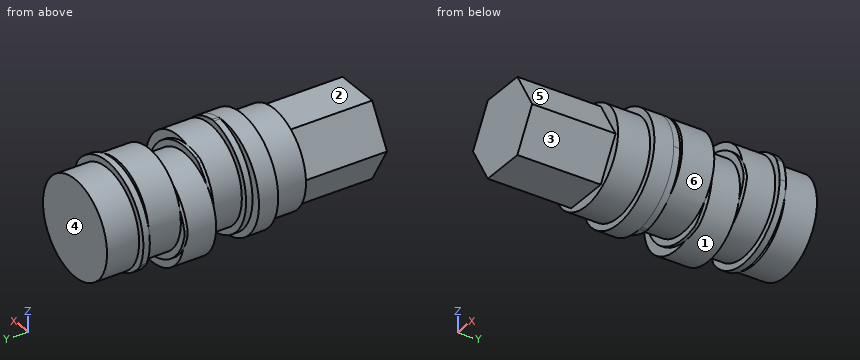
from build123d import *

# Parameters (mm, degrees)
BOSS_EXTRUDE1_DEPTH  = 13
SKETCH5_R            = 7.5
BOSS_EXTRUDE2_DEPTH  = 8
BOSS_EXTRUDE3_DEPTH  = 1
SKETCH7_R            = 7.5
BOSS_EXTRUDE4_DEPTH  = 5
BOSS_EXTRUDE5_DEPTH  = 0.5
SKETCH9_R            = 7.5
BOSS_EXTRUDE6_DEPTH  = 5
BOSS_EXTRUDE7_DEPTH  = 0.5
SKETCH12_R           = 7.5
BOSS_EXTRUDE8_DEPTH  = 5
BOSS_EXTRUDE9_DEPTH  = 1
SKETCH14_R           = 7.5
BOSS_EXTRUDE10_DEPTH = 5
FILLET1_R            = 2
BOSS_EXTRUDE11_START = 3
SKETCH15_R           = 8.5
BOSS_EXTRUDE11_DEPTH = 3


with BuildPart() as part:
    # Sketch4 → Boss-Extrude1 (new body)
    with BuildSketch(Plane(origin=(0, 0, 0), x_dir=(1, 0, 0), z_dir=(0, 1, 0))):
        Polygon((-3.464101615, 6), (-6.92820323, 0), (-3.464101615, -6), (3.464101615, -6), (6.92820323, 0), (3.464101615, 6), align=None)
    extrude(amount=BOSS_EXTRUDE1_DEPTH)

    # Sketch5 → Boss-Extrude2 (add)
    with BuildSketch(Plane(origin=(0, 13, 0), x_dir=(1, 0, 0), z_dir=(0, 1, 0))):
        with Locations(Location((0, 0, 0), (0, 0, 270))):
            Circle(SKETCH5_R)
    extrude(amount=BOSS_EXTRUDE2_DEPTH)

    # Sketch6 → Boss-Extrude3 (add)
    with BuildSketch(Plane(origin=(0, 21, 0), x_dir=(1, 0, 0), z_dir=(0, 1, 0))):
        with BuildLine():
            ThreePointArc((0.75, -8.466847111), (6.269968102, -5.739120142), (8.5, 0))
            ThreePointArc((8.5, 0), (6.269968102, 5.739120142), (0.75, 8.466847111))
            ThreePointArc((0.75, 8.466847111), (-7, 0), (0.75, -8.466847111))
        make_face()
    extrude(amount=BOSS_EXTRUDE3_DEPTH)

    # Sketch7 → Boss-Extrude4 (add)
    with BuildSketch(Plane(origin=(0, 22, 0), x_dir=(1, 0, 0), z_dir=(0, 1, 0))):
        with Locations(Location((1.5, 0, 0), (0, 0, 52.330113036))):
            Circle(SKETCH7_R)
    extrude(amount=BOSS_EXTRUDE4_DEPTH)

    # Sketch8 → Boss-Extrude5 (add)
    with BuildSketch(Plane(origin=(0, 27, 0), x_dir=(1, 0, 0), z_dir=(0, 1, 0))):
        with BuildLine():
            ThreePointArc((7.75, 1.299038106), (6.915283179, 4.972379062), (4.575074404, 7.924261316))
            ThreePointArc((4.575074404, 7.924261316), (-5.861215932, 4.25), (-3.825074404, -6.625223211))
            ThreePointArc((-3.825074404, -6.625223211), (4.051659482, -5.714810069), (7.75, 1.299038106))
        make_face()
    extrude(amount=BOSS_EXTRUDE5_DEPTH)

    # Sketch9 → Boss-Extrude6 (add)
    with BuildSketch(Plane(origin=(0, 27.5, 0), x_dir=(1, 0, 0), z_dir=(0, 1, 0))):
        with Locations(Location((-0.75, 1.299038106, 0), (0, 0, 73.730489259))):
            Circle(SKETCH9_R)
    extrude(amount=BOSS_EXTRUDE6_DEPTH)

    # Sketch11 → Boss-Extrude7 (add)
    with BuildSketch(Plane(origin=(0, 32.5, 0), x_dir=(1, 0, 0), z_dir=(0, 1, 0))):
        with BuildLine():
            ThreePointArc((7.650148808, 0), (-0.75, 7.200961894), (-9.150148808, 0))
            ThreePointArc((-9.150148808, 0), (-0.75, -7.200961894), (7.650148808, 0))
        make_face()
    extrude(amount=BOSS_EXTRUDE7_DEPTH)

    # Sketch12 → Boss-Extrude8 (add)
    with BuildSketch(Plane(origin=(0, 33, 0), x_dir=(1, 0, 0), z_dir=(0, 1, 0))):
        with Locations(Location((-0.75, -1.299038106, 0), (0, 0, 193.730489259))):
            Circle(SKETCH12_R)
    extrude(amount=BOSS_EXTRUDE8_DEPTH)

    # Sketch13 → Boss-Extrude9 (add)
    with BuildSketch(Plane(origin=(0, 38, 0), x_dir=(1, 0, 0), z_dir=(0, 1, 0))):
        with BuildLine():
            ThreePointArc((6.957504688, -4.882942608), (7.549511728, -3.134277893), (7.75, -1.299038106))
            ThreePointArc((7.75, -1.299038106), (1.810391586, 6.806169783), (-7.707504688, 3.583904503))
            ThreePointArc((-7.707504688, 3.583904503), (-4.25, -7.361215932), (6.957504688, -4.882942608))
        make_face()
    extrude(amount=BOSS_EXTRUDE9_DEPTH)

    # Sketch14 → Boss-Extrude10 (add)
    with BuildSketch(Plane(origin=(0, 39, 0), x_dir=(1, 0, 0), z_dir=(0, 1, 0))):
        with Locations(Location((0, 0, 0), (0, 0, 127.669886964))):
            Circle(SKETCH14_R)
    extrude(amount=BOSS_EXTRUDE10_DEPTH)

    # Fillet1
    fillet1_edges = [part.edges().sort_by_distance(p)[0] for p in [
        (0.75, 21.5, -8.466847111),
        (0.75, 21.5, 8.466847111),
        (-3.825074404, 27.25, 6.625223211),
        (4.575074404, 27.25, -7.924261316),
        (7.650148808, 32.75, 0),
        (-9.150148808, 32.75, 0),
        (-7.707504688, 38.5, -3.583904503),
        (6.957504688, 38.5, 4.882942608),
    ]]
    fillet(fillet1_edges, radius=FILLET1_R)

    # Sketch15 → Boss-Extrude11 (add)
    with BuildSketch(Plane.XZ.offset(-21).offset(BOSS_EXTRUDE11_START)):
        with Locations(Location((0, 0, 0), (0, 0, 270))):
            Circle(SKETCH15_R)
    extrude(amount=-BOSS_EXTRUDE11_DEPTH)


solid = part.part
Verification items for the finished model (mm, model axes). Face numbers are marked on the shaded views. A direction names the side the tool comes from. Round coordinates to 2 decimals unless told otherwise and drop trailing zeros. Order: outer loops, then holes, each group sorted by start corner. A loop starts at its lowest first (then second) coordinate and runs counter-clockwise, first axis right, second up.
1. Access from +Z, -Z, +X, -X, +Y, -Y to the whole of each face (thin tool, end or side, straight path). Record for the marked faces 1, 2 and 3.
Final values:
face 1: none
face 2: +Z, +X, -X, -Y
face 3: -Z, +X, -Y
2. Thickness scan on L1, parallel to Y at x = 4.75, z = -7; L2, parallel to Y at x = -4.5, z = -5; L3, parallel to Z at x = 1, y = 3.5. Record the ranges inside material, lowest first.
Final values:
L1: y = 18 to 22, 27 to 27.5
L2: y = 13 to 22, 27 to 44
L3: z = -6 to 6
3. Section check A-A on y = 6. Record the cut outline in (x, z), then the cut area to 3 significant figures.
Final values:
outline: (-6.93, 0) - (-3.46, -6) - (3.46, -6) - (6.93, 0) - (3.46, 6) - (-3.46, 6) - close
area: 125 mm2
4. Go/stop test with flat-tipped pins: P1, Ø6, axis at x = -2, z = 0, coming from the -Y side; P2, Ø1.5, axis at x = -4.5, y = 6.5, coming from the -Z side; P3, Ø10, axis at y = 9, z = 1.5, coming from the +X side; P4, Ø5.5, axis at x = 1, y = 9, coming from the +Z side. Record where each tip stops, or that it passes through.
Final values:
P1: stops at y = 0
P2: stops at z = -5.5
P3: stops at x = 7.5
P4: stops at z = 6
5. Release check for a two-part mould opening along Y. For the marked faces 4, 5 and 6 record: +Y half, -Y half, draft (parallel to the pull), parting line (faces both ways), or undercut.
Final values:
face 4: +Y half
face 5: draft
face 6: undercut
6. Section check B-B on y = 31.5. Record the cut outline in (x, z), then the cut area to 3 significant figures.
Final values:
outline: circle Ø15 at (-0.75, -1.3)
area: 177 mm2
